from build123d import *

# Parameters (mm, degrees)
EXTRUSION1_DEPTH = 20
ESQUISSE2_R      = 1.5
EXTRUSION2_DEPTH = 42.382154348
ESQUISSE4_R      = 3
EXTRUSION3_DEPTH = 32.911544508
ESQUISSE5_R      = 3.11
EXTRUSION4_DEPTH = 33.803912463


with BuildPart() as part:
    # Esquisse1 → Extrusion1 (new body)
    with BuildSketch(Plane.XY):
        Polygon((-31.14855853, 3.383843017), (-29.64855853, 3.383843017), (-29.64855853, -15.116156983), (-12.64855853, -15.116156983), (-12.64855853, 3.383843017), (-11.14855853, 3.383843017), (-11.14855853, -16.616156983), (-31.14855853, -16.616156983), align=None)
    extrude(amount=EXTRUSION1_DEPTH)

    # Esquisse2 → Extrusion2 (cut, through all)
    with BuildSketch(Plane(origin=(0, -15.116156983, 0), x_dir=(-1, 0, 0), z_dir=(0, 1, 0))):
        with Locations((26.14855853, 13)):
            Circle(ESQUISSE2_R)
        with Locations((16.14855853, 7)):
            Circle(ESQUISSE2_R)
    extrude(amount=-EXTRUSION2_DEPTH, mode=Mode.SUBTRACT)

    # Esquisse4 → Extrusion3 (cut, through all)
    with BuildSketch(Plane(origin=(-29.64855853, 0, 0), x_dir=(0, 0, -1), z_dir=(1, 0, 0))):
        with Locations(Location((-5, -2.616156983, 0), (0, 0, 90))):
            Circle(ESQUISSE4_R)
    extrude(amount=-EXTRUSION3_DEPTH, mode=Mode.SUBTRACT)

    # Esquisse5 → Extrusion4 (cut, through all)
    with BuildSketch(Plane.ZY.offset(31.14855853)):
        with Locations((15.5, -2.616156983)):
            Circle(ESQUISSE5_R)
    extrude(amount=-EXTRUSION4_DEPTH, mode=Mode.SUBTRACT)


solid = part.part
Source: CAD feature listing. Evaluate the final solid. Frame: model axes, mm. A direction names the side the tool comes from. Give positions to 0.01 mm unless a question says otherwise; leave off trailing zeros. Write each loop counter-clockwise with the first axis right and the second up, starting at its lowest first coordinate (ties: lowest second). Pieces come first, ordered by that corner, then holes. Notation, with made-up numbers: M 80,17.5 L 118,17.5 A10 ccw 118,33.5 Z; hole C -30,-10.5 d3. An arc over 180 degrees is marked long. Return JSON: item names as keys, results as strings. Group by question number.
1) Cut plane D-D, the plane y = -3.5. Output: boundary loops of the cut face in (x, z), plus the area to 3 significant figures.
2) Material intervals for line 1 along X through (y, z) = (-13.75, 12); line 2 along Y through (x, z) = (-13, 4.5); line 3 along X through (y, z) = (-4.5, 2.75), sorted ascending. Write a range as [from, to].
3) Pin query (flat end, axial travel): P1, Ø2.5, axis at x = -16.15, z = 7, coming from the +Y side. Return the tip coordinate at first contact, or that it passes through.
4) Cut plane A-A, the plane z = 15.5. Output: boundary loops of the cut face in (x, y), plus the area to 3 significant figures.
5) Set-up query: faces 1 (the face through (-31.149, -7, 10)), 2 (the face through (-30.388, -3.266, 2.071)), 3 (the face through (-12.649, -6, 10)). Return all of +Z, -Z, +X, -X, +Y, -Y with unobstructed straight access to the full face (end or side cutting, diameter ignored); none if empty.
6) Cut plane B-B, the plane y = -12.75. Output: boundary loops of the cut face in (x, z).
7) Pull-direction query (Y, two-part tool) for faces 4 (the face through (-17.534, -15.856, 6.425)), 5 (the face through (-30, 3.384, 10)), 6 (the face through (-11.91, -3.81, 18.37)); classes: pulls with the +Y half, pulls with the -Y half, needs draft (parallel to the pull), parting line crosses it, or undercut.
8) Cut plane C-C, the plane z = 13. Output: boundary loops of the cut face in (x, y), plus the area to 3 significant figures.
Recorded:
{
 "1": {"outline": "M -31.15,0 L -29.65,0 L -29.65,2.13 L -31.15,2.13 Z; M -31.15,7.87 L -29.65,7.87 L -29.65,12.52 L -31.15,12.52 Z; M -31.15,18.48 L -29.65,18.48 L -29.65,20 L -31.15,20 Z; M -12.65,0 L -11.15,0 L -11.15,12.52 L -12.65,12.52 Z; M -12.65,18.48 L -11.15,18.48 L -11.15,20 L -12.65,20 Z", "area": "33.5 mm²"},
 "2": {"line 1": "x = [-31.15, -29.65], [-12.65, -11.15]", "line 2": "y = [-16.62, -15.12]", "line 3": "x = [-12.65, -11.15]"},
 "3": {"P1": "passes through"},
 "4": {"outline": "M -31.15,-16.62 L -11.15,-16.62 L -11.15,-5.73 L -12.65,-5.73 L -12.65,-15.12 L -29.65,-15.12 L -29.65,-5.73 L -31.15,-5.73 Z; M -31.15,0.49 L -29.65,0.49 L -29.65,3.38 L -31.15,3.38 Z; M -12.65,0.49 L -11.15,0.49 L -11.15,3.38 L -12.65,3.38 Z", "area": "66.8 mm²"},
 "5": {"face 1": "+Z, -Z, -X, +Y, -Y", "face 2": "-X", "face 3": "+Z, -Z, +Y"},
 "6": {"outline": "M -31.15,0 L -29.65,0 L -29.65,20 L -31.15,20 Z; M -12.65,0 L -11.15,0 L -11.15,20 L -12.65,20 Z"},
 "7": {"face 4": "needs draft", "face 5": "pulls with the +Y half", "face 6": "undercut"},
 "8": {"outline": "M -31.15,-16.62 L -27.65,-16.62 L -27.65,-15.12 L -29.65,-15.12 L -29.65,-4.47 L -31.15,-4.47 Z; M -31.15,-0.77 L -29.65,-0.77 L -29.65,3.38 L -31.15,3.38 Z; M -24.65,-16.62 L -11.15,-16.62 L -11.15,-4.47 L -12.65,-4.47 L -12.65,-15.12 L -24.65,-15.12 Z; M -12.65,-0.77 L -11.15,-0.77 L -11.15,3.38 L -12.65,3.38 Z", "area": "69.9 mm²"}
}
